The listing builds one solid part. Answer for the finished solid, in the listing's coordinates (mm). Coordinates: 2 decimals unless noted, no trailing zeros. Loops run counter-clockwise (first coordinate to the right, second up) from the corner with the lowest first, then second, coordinate; pieces in that order, holes last. Notation, with made-up numbers: M 24.5,-8.5 L 68.5,-8.5 A30 cw 68.5,14.5 Z; hole C 46,-8.5 d5. An arc over 180 degrees is marked long. Answer as a JSON object with one key per item and string values. Group by question number.
1. A cutting plane is placed at B-B on x = 79.5. Give the vertices of the cut face in (y, z), and give its area (3 significant figures).
2. A cutting plane is placed at C-C on y = 36.5. Give the vertices of the cut face in (x, z).
3. A cutting plane is placed at A-A on z = 2.45. Give the vertices of the cut face in (x, y).
4. Straight lines are drawn through the part: L1, parallel to Y at x = 73, z = 0.15; L2, parallel to Y at x = 90, z = 1.35; L3, parallel to X at y = 14, z = 1.1. For each, find the intervals that lie inside material, in ascending order.
5. Given pin 1 (1 mm diameter, centred on y = 41, z = 2.5, fed in from +X); pin 2 (1.5 mm diameter, centred on y = 30, z = 2.5, fed in from +X); pin 3 (1.5 mm diameter, centred on x = 49.5, z = 1, fed in from +Y), each flat-ended and moving along its own axis, determine where each tip first touches the part or whether it passes through.
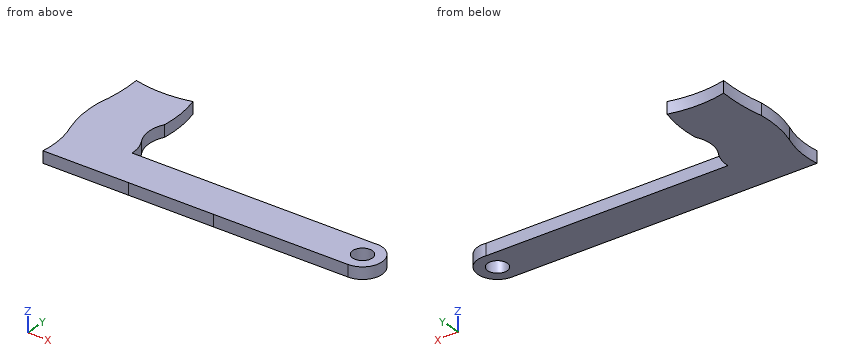
from build123d import *

# Parameters (mm, degrees)
MODEL_R                 = 2.5
SALIENTE_EXTRUIR1_DEPTH = 3


with BuildPart() as part:
    # Model → Saliente-Extruir1 (new body)
    with BuildSketch(Plane.XY):
        with BuildLine():
            Line((11.080118073, 12.100032616), (32.626217211, 12.100005802))
            Line((32.626217211, 12.100005802), (54.087474295, 12.099999973))
            Line((54.087474295, 12.099999973), (88.080119434, 12.099990741))
            ThreePointArc((88.080119434, 12.099990741), (93.069612737, 17.423981681), (87.43349937, 22.058002513))
            Line((87.43349937, 22.058002513), (26.334882576, 22.058035741))
            ThreePointArc((26.334882576, 22.058035741), (26.077271745, 24.671051179), (25.080126231, 27.100025003))
            ThreePointArc((25.080126231, 27.100025003), (24.017870658, 31.10002558), (25.080130581, 35.100025003))
            ThreePointArc((25.080130581, 35.100025003), (25.229028906, 40.534712367), (24.350613381, 45.900006732))
            ThreePointArc((24.350613381, 45.900006732), (17.215374003, 45.022517475), (10.080135103, 45.900010617))
            ThreePointArc((10.080135103, 45.900010617), (9.999432675, 39.964488004), (9.080130038, 34.100033704))
            ThreePointArc((9.080130038, 34.100033704), (9.035519695, 28.550523972), (10.080124055, 23.10003316))
            ThreePointArc((10.080124055, 23.10003316), (11.257202039, 17.661585333), (11.080118073, 12.100032616))
        make_face()
        with Locations((88.080120792, 17.099990741)):
            Circle(MODEL_R, mode=Mode.SUBTRACT)
    extrude(amount=SALIENTE_EXTRUIR1_DEPTH)


solid = part.part
From the geometry:
{
 "1": {"outline": "M 12.1,0 L 22.06,0 L 22.06,3 L 12.1,3 Z", "area": "29.9 mm²"},
 "2": {"outline": "M 9.56,0 L 25.22,0 L 25.22,3 L 9.56,3 Z"},
 "3": {"outline": "M 9.08,34.1 A28.16 ccw 10.08,23.1 A22.77 cw 11.08,12.1 L 32.63,12.1 L 88.08,12.1 A5 ccw long 87.43,22.06 L 26.33,22.06 A9.05 ccw 25.08,27.1 A8.06 cw 25.08,35.1 A28.71 ccw 24.35,45.9 A29.45 cw 10.08,45.9 A41.87 cw Z; hole C 88.08,17.1 d5"},
 "4": {"L1": "y = 12.1 to 22.06", "L2": "y = 12.48 to 15.5, 18.7 to 21.72", "L3": "x = 11.29 to 92"},
 "5": {"pin 1": "stops at x = 25.23", "pin 2": "stops at x = 24.23", "pin 3": "stops at y = 22.06"}
}
